```python
from build123d import *

# Parameters (mm, degrees)
CHANFREIN1_SIZE         = 0.5
ENL_V_MAT_EXTRU_1_DEPTH = 1.8


with BuildPart() as part:
    # Esquisse1 → Révolution1 (revolve)
    with BuildSketch(Plane.XY):
        Polygon((0, 0), (0, 4), (0.3, 4), (2.3, 2), (6, 2), (6, 0), align=None)
    revolve(axis=Axis((6, 0, 0), (-1, 0, 0)))

    # Chanfrein1
    chanfrein1_edges = [part.edges().sort_by_distance(p)[0] for p in [
        (6, -2, 0),
    ]]
    chamfer(chanfrein1_edges, length=CHANFREIN1_SIZE)

    # Esquisse2 → Enlèv. mat.-Extru.1 (cut)
    with BuildSketch(Plane.ZY):
        Polygon((0, 1.443375673), (-1.25, 0.721687836), (-1.25, -0.721687836), (0, -1.443375673), (1.25, -0.721687836), (1.25, 0.721687836), align=None)
    extrude(amount=-ENL_V_MAT_EXTRU_1_DEPTH, mode=Mode.SUBTRACT)


solid = part.part
```
Part model, mm, in its own coordinate system. A direction names the side the tool comes from. Coordinates: 2 decimals unless noted, no trailing zeros. Write each loop counter-clockwise with the first axis right and the second up, starting at its lowest first coordinate (ties: lowest second). Pieces come first, ordered by that corner, then holes.
Item 1: Mould opens along Y. For faces 1 (the face through (4, 0, 2)), 2 (the face through (1, 0, -1.25)), 3 (the face through (0, -2, 0)), 4 (the face through (0.89, -1.08, -0.63)) say: released by +Y, released by -Y, zero draft, split by the parting line, or undercut.
Item 2: Which spindle directions (+Z, -Z, +X, -X, +Y, -Y) get a long thin tool onto all of the face, cutting with end or side? Do faces 5 (the face through (6, 0, 0)), 6 (the face through (0.887, 1.088, -0.616)). Say none if no direction does.
Item 3: Probe line 1 (Z direction, x = 1.7, y = -1); line 2 (Z direction, x = 4.05, y = 0). List the from-to ranges inside material, lowest first.
Item 4: Slice it at B-B (y = 0). Write the cut outline in (x, z).
Item 5: Pin check, flat tips, straight feed: pin 1 (2 mm diameter, centred on x = 2, y = 1, fed in from -Z); pin 2 (1 mm diameter, centred on x = 3, y = 2, fed in from -Z); pin 3 (0.7 mm diameter, centred on x = 1, y = 0, fed in from +Z). Stop position of each tip, or through.
Item 6: Slice it at A-A (x = 1.1). Write the cut outline in (y, z).
Item 7: Slice it at C-C (x = 3.3). Write the cut outline in (y, z).
Results found:
1. face 1: split by the parting line
1. face 2: undercut
1. face 3: zero draft
1. face 4: undercut
2. face 5: +Z, -Z, +X, +Y, -Y
2. face 6: -X
3. line 1: z = -2.4 to -0.77, 0.77 to 2.4
3. line 2: z = -2 to 2
4. outline: (0, -4) - (0.3, -4) - (2.3, -2) - (5.5, -2) - (6, -1.5) - (6, 1.5) - (5.5, 2) - (2.3, 2) - (0.3, 4) - (0, 4) - (0, 1.25) - (1.8, 1.25) - (1.8, -1.25) - (0, -1.25) - close
5. pin 1: stops at z = -3.18
5. pin 2: stops at z = -1.32
5. pin 3: stops at z = 3.65
6. outline: circle Ø6.4 at (0, 0); hole (-1.44, 0) - (-0.72, -1.25) - (0.72, -1.25) - (1.44, 0) - (0.72, 1.25) - (-0.72, 1.25) - close
7. outline: circle Ø4 at (0, 0)
